Here's how the part is built. I have some questions about the finished solid (model axes, mm). A direction names the side the tool comes from. Give positions to 0.01 mm unless a question says otherwise; leave off trailing zeros. Write each loop counter-clockwise with the first axis right and the second up, starting at its lowest first coordinate (ties: lowest second). Pieces come first, ordered by that corner, then holes. Notation, with made-up numbers: (-13.75, 21.5) -> (4.25, 21.5) arc R19 ccw to (4.25, 42.5) -> close; hole circle Ø9 at (71, 26). An arc over 180 degrees is marked (long way). Put each result on its own line as item: value. Start each with the question number.
Autodesk Inventor part; units mm, degrees
ref_plane "YZ Plane" through (0, 0, 0) normal (1, 0, 0) x (0, 1, 0)
ref_plane "XZ Plane" through (0, 0, 0) normal (0, 1, 0) x (-1, 0, 0)
ref_plane "XY Plane" through (0, 0, 0) normal (0, 0, 1) x (1, 0, 0)
sketch "Sketch1" plane through (0, 0, 0) normal (0, 0, 1) x (1, 0, 0)
  line L0 (0, 0) -> (9, 0)
  line L1 (9, 0) -> (9, 13.8)
  line L2 (9, 13.8) -> (0, 13.8)
  line L3 (0, 13.8) -> (0, 0)
  dimension "d0" = 9
  dimension "d1" = 13.8
extrude "Extrusion1" add sketch "Sketch1" along normal blind 8.9
sketch "Sketch2" plane through (0, 0, 8.9) normal (0, 0, 1) x (1, 0, 0)
  line L0 (-0.75, 14.4) -> (9.75, 14.4)
  line L1 (9.75, 14.4) -> (9.75, -0.6)
  line L2 (9.75, -0.6) -> (-0.75, -0.6)
  line L3 (-0.75, -0.6) -> (-0.75, 14.4)
  line L4 (9, 13.8) -> (0, 13.8)
  line L5 (0, 13.8) -> (0, 0)
  dimension "d4" = 10.5
  dimension "d5" = 15
  dimension "d6" = 0.6
  dimension "d7" = 0.75
extrude "Extrusion2" add sketch "Sketch2" along normal blind 1.6
sketch "Sketch3" plane through (0, 0, 10.5) normal (0, 0, 1) x (1, 0, 0)
  line L0 (1.2958, 12.4644) -> (7.672, 12.4644)
  line L1 (7.672, 12.4644) -> (7.672, 1.1518)
  line L2 (7.672, 1.1518) -> (1.2958, 1.1518)
  line L3 (1.2958, 1.1518) -> (1.2958, 12.4644)
  point P0 (0, 0)
extrude "Extrusion3" add sketch "Sketch3" along normal blind 2
chamfer "Chamfer1" distance 11.25 angle 10 1 edges at (4.4839, 1.1518, 12.5) measured on face at (3.4212, 8.6935, 12.5)
sketch "Sketch4" plane through (0, 0, 0) normal (0, 0, -1) x (-1, 0, 0)
  line L0 (-6.4, 1.7) -> (-2.6, 1.7)
  line L1 (-2.6, 1.7) -> (-2.6, 1.3)
  line L2 (-2.6, 1.3) -> (-6.4, 1.3)
  line L3 (-6.4, 1.3) -> (-6.4, 1.7)
  line L4 (-9, 0) -> (-9, 13.8)
  line L5 (0, 0) -> (-9, 0)
  point P0 (-6.4, 1.5)
  dimension "d15" = 3.8
  dimension "d16" = 0.4
  dimension "d17" = 2.6
  dimension "d18" = 1.3
extrude "Extrusion4" add sketch "Sketch4" along normal blind 7.3
fillet "Fillet1" radius 1 2 edges at (2.6, 1.5, -7.3) (6.4, 1.5, -7.3)
sketch "Sketch5" plane through (2.6, 1.7, 0) normal (0, 1, 0) x (1, 0, 0)
  line L0 (2.2682, 5.9403) -> (1.4834, 5.9403)
  line L1 (1.2834, 5.7403) -> (1.2834, 3.5404)
  line L2 (1.4834, 3.3404) -> (2.2682, 3.3404)
  line L3 (2.4682, 3.5404) -> (2.4682, 5.7403)
  arc A0 (2.4682, 5.7403) -> (2.2682, 5.9403) centre (2.2682, 5.7403) ccw
  arc A1 (1.4834, 5.9403) -> (1.2834, 5.7403) centre (1.4834, 5.7403) ccw
  arc A2 (2.2682, 3.3404) -> (2.4682, 3.5404) centre (2.2682, 3.5404) ccw
  arc A3 (1.2834, 3.5404) -> (1.4834, 3.3404) centre (1.4834, 3.5404) ccw
  point P0 (-2.6, 0)
  dimension "d22" = 0.2
extrude "Extrusion5" cut sketch "Sketch5" against normal blind 7.3
pattern_linear "Rectangular Pattern1" count 2 spacing 4.6 along (0, 1, 0) of "Extrusion4", "Extrusion5", "Fillet1"
properties part number "rocker_switch"
1) Thinking about a two-plate mould opening in Y: for faces 1 (the flat face through (5, 1.7, -3)), 2 (the flat face through (5, 13.8, 4)), 3 (the flat face through (7.672, 8, 11)), 4 (the flat face through (4, 5.9, -3)), which applies, released by +Y, released by -Y, zero draft, split by the parting line, or undercut?
2) I need wall thicknesses on probe 1 along X at (y, z) = (1.5, -5.5); probe 2 along Y at (x, z) = (5.5, -0.25); probe 3 along Y at (x, z) = (2.75, 5.25). Which ranges of each line are inside material? Lowest first, please.
3) I'm going to push flat-ended pins straight in: pin 1 Ø1 at (x, z) = (4, -1) entering from +Y; pin 2 Ø1.5 at (x, z) = (3, 1.5) entering from +Y; pin 3 Ø8 at (y, z) = (4.5, -3) entering from +X. Where does each tip first touch, or does it pass through?
4) Which directions (+Z, -Z, +X, -X, +Y, -Y) give clear straight access to the entire face, cutting with the end or side of a thin tool? Please do faces 5 (the flat face through (9, 7, 4)), 6 (the flat face through (1.296, 8, 11)), 7 (the flat face through (4, 12.464, 11)), 8 (the cylindrical face through (2.885, 6.097, -6.999)), 9 (the flat face through (4, 0, 4)).
5) I want a section at A-A, the plane x = 8. Write out the boundary of the cut face in (y, z).
6) I want a section at C-C, the plane z = 7. Write out the boundary of the cut face in (x, y), and give its area (3 significant figures).
7) I want a section at B-B, the plane y = 8.75. Write out the boundary of the cut face in (x, z), and give its area (3 significant figures).
Established:
1. face 1: undercut
1. face 2: released by +Y
1. face 3: zero draft
1. face 4: undercut
2. probe 1: x = 2.6 to 3.88, 5.07 to 6.4
2. probe 2: y = 1.3 to 1.7, 5.9 to 6.3
2. probe 3: y = 0 to 13.8
3. pin 1: stops at y = 6.3
3. pin 2: stops at y = 13.8
3. pin 3: stops at x = 9
4. face 5: -Z, +X, +Y, -Y
4. face 6: +Z, -X, +Y, -Y
4. face 7: +Z, +X, -X, +Y
4. face 8: -Z, -X, +Y, -Y
4. face 9: -Z, +X, -X, -Y
5. outline: (-0.6, 8.9) -> (0, 8.9) -> (0, 0) -> (13.8, 0) -> (13.8, 8.9) -> (14.4, 8.9) -> (14.4, 10.5) -> (-0.6, 10.5) -> close
6. outline: (0, 0) -> (9, 0) -> (9, 13.8) -> (0, 13.8) -> close
6. area: 124 mm2
7. outline: (-0.75, 8.9) -> (0, 8.9) -> (0, 0) -> (9, 0) -> (9, 8.9) -> (9.75, 8.9) -> (9.75, 10.5) -> (7.67, 10.5) -> (7.67, 11.86) -> (1.3, 11.86) -> (1.3, 10.5) -> (-0.75, 10.5) -> close
7. area: 106 mm2
